from build123d import *

# Parameters (mm, degrees)
F1_DEPTH = 75
F2_W     = 2.844389
F2_H     = 55
F3_DEPTH = 12
F5_DEPTH = 12
F6_W     = 3
F6_H     = 55
F6_H_2   = 10
F7_DEPTH = 12


with BuildPart() as f1:
    # F0 (on Right) → F1 (new body, symmetric)
    with BuildSketch(Plane.YZ):
        Polygon((-6, -34), (6, -34), (6, 34), (-6, 34), (-6, 24), (-3, 24), (-3, 21), (-6, 21), align=None)
    extrude(amount=F1_DEPTH, both=True)

    # F2 (on face) → F3 (cut)
    with BuildSketch(Plane.YZ.offset(75)):
        with Locations((-4.577806, -6.5)):
            Rectangle(F2_W, F2_H)
    extrude(amount=-F3_DEPTH, mode=Mode.SUBTRACT)

    # F4 (on face) → F5 (cut)
    with BuildSketch(Plane.YZ.offset(75)):
        Polygon((-6, 24), (-3.098777, 24), (-3, 34), (-6, 34), align=None)
    extrude(amount=-F5_DEPTH, mode=Mode.SUBTRACT)

    # F6 (on face) → F7 (cut)
    with BuildSketch(Plane(origin=(-75, 0, 0), x_dir=(0, -1, 0), z_dir=(-1, 0, 0))):
        with Locations((4.5, -6.5)):
            Rectangle(F6_W, F6_H)
        with Locations((4.5, 29)):
            Rectangle(F6_W, F6_H_2)
    extrude(amount=-F7_DEPTH, mode=Mode.SUBTRACT)


solid = f1.part
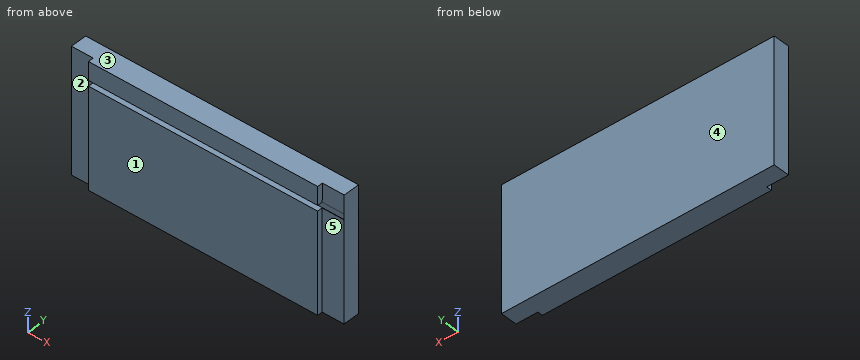
Work out the finished part from the listing and answer in its coordinate system (mm). Face numbers are marked on the shaded views. A direction names the side the tool comes from. Give positions to 0.01 mm unless a question says otherwise; leave off trailing zeros. Order: outer loops, then holes, each group sorted by start corner. A loop starts at its lowest first (then second) coordinate and runs counter-clockwise, first axis right, second up. Notation, with made-up numbers: (25, 30) - (69, 30) arc R21 ccw to (69, 39) - close; hole circle Ø10 at (56, 70). An arc over 180 degrees is marked (long way). Answer as CSV lines item,"result". Start each with the question number.
Q1. The mould has two halves that part along Z. Classify the marked faces 1, 2 and 3: +Z half, -Z half, draft (parallel to the pull), parting line (faces both ways), or undercut.
Q2. The part is cut by section A-A (z = -17.5). Write down the section's boundary in (x, y), then the cut area to 3 significant figures.
Q3. Find the intervals of material crossed by L1, parallel to Z at x = 59, y = -3.5; L2, parallel to X at y = -4, z = 5; L3, parallel to Y at x = -27, z = 23, in increasing order. Write a range as [from, to].
Q4. For the marked faces 4 and 5, determine the directions among +Z, -Z, +X, -X, +Y, -Y from which every point of the face is accessible in a straight line to the end or side of a thin tool.
Q5. The part is cut by section B-B (z = 27). Write down the section's boundary in (x, y).
Q6. Given pin 1 Ø9.5 at (x, z) = (70, -8.5) entering from -Y; pin 2 Ø0.9 at (y, z) = (-4, 29) entering from +X; pin 3 Ø2.5 at (y, z) = (-4.5, 28) entering from -X, each flat-ended and moving along its own axis, determine where each tip first touches the part or whether it passes through.
Check result:
1,face 1,"draft"
1,face 2,"undercut"
1,face 3,"+Z half"
2,outline,"(-75, -3) - (-63, -3) - (-63, -6) - (63, -6) - (63, -3.16) - (75, -3.16) - (75, 6) - (-75, 6) - close"
2,area,"1,730 mm²"
3,L1,"z = [-34, 21], [24, 34]"
3,L2,"x = [-63, 63]"
3,L3,"y = [-3, 6]"
4,face 4,"+Z, -Z, +X, -X, +Y"
4,face 5,"+Z, -Z, +X, -Y"
5,outline,"(-75, -3) - (-63, -3) - (-63, -6) - (63, -6) - (63, -3.07) - (75, -3.07) - (75, 6) - (-75, 6) - close"
6,pin 1,"stops at y = -3.16"
6,pin 2,"stops at x = 63"
6,pin 3,"stops at x = -63"
